Design review of the part built by this model. Coordinates are the model's own, in mm. Face numbers are marked on the shaded views. A direction names the side the tool comes from. Coordinates: 2 decimals unless noted, no trailing zeros. Loops run counter-clockwise (first coordinate to the right, second up) from the corner with the lowest first, then second, coordinate; pieces in that order, holes last. Notation, with made-up numbers: (27, 58) -> (48, 58) arc R12 ccw to (48, 81) -> close; hole circle Ø11 at (31, 33.25). An arc over 180 degrees is marked (long way). Answer in a Markdown table with one row per item.
```python
from build123d import *

# Parameters (mm, degrees)
BOSS_EXTRUDE1_DEPTH     = 3.25
SKETCH2_R               = 3.76
BOSS_EXTRUDE2_DEPTH     = 1.75
CUT_EXTRUDE1_DEPTH      = 8.895146188
CUT_EXTRUDE1_DEPTH_BACK = 8.895146188
SKETCH3_R               = 2.5


with BuildPart() as part:
    # Sketch1 → Boss-Extrude1 (new body)
    with BuildSketch(Plane(origin=(0, 0, 0), x_dir=(1, 0, 0), z_dir=(0, 1, 0))):
        Polygon((4, -2.309401077), (0, -4.618802154), (-4, -2.309401077), (-4, 2.309401077), (0, 4.618802154), (4, 2.309401077), align=None)
    extrude(amount=-BOSS_EXTRUDE1_DEPTH)

    # Sketch2 → Boss-Extrude2 (add)
    with BuildSketch(Plane(origin=(0, -3.25, 0), x_dir=(1, 0, 0), z_dir=(0, 1, 0))):
        with Locations(Location((0, 0, 0), (0, 0, 270))):
            Circle(SKETCH2_R)
    extrude(amount=-BOSS_EXTRUDE2_DEPTH)

    # Sketch3 → Cut-Extrude1 (cut, two sides: drawn at the far end of the back side and taken through both)
    with BuildSketch(Plane(origin=(0, 0, 0), x_dir=(1, 0, 0), z_dir=(0, 1, 0)).offset(-CUT_EXTRUDE1_DEPTH_BACK)):
        with Locations(Location((0, 0, 0), (0, 0, 270))):
            Circle(SKETCH3_R)
    extrude(amount=CUT_EXTRUDE1_DEPTH + CUT_EXTRUDE1_DEPTH_BACK, mode=Mode.SUBTRACT)


solid = part.part
```
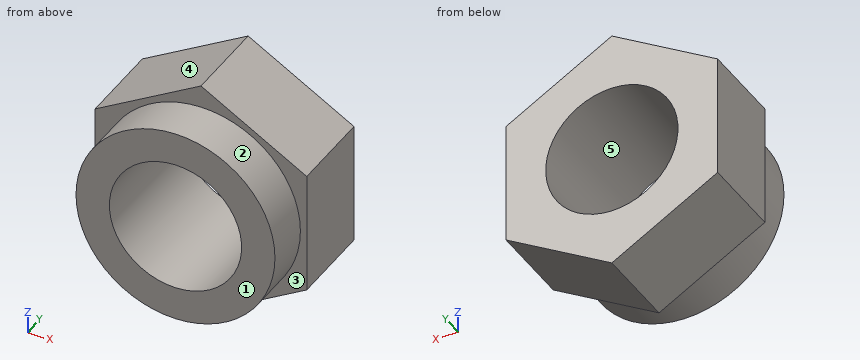
(1) To check wall thickness, follow probe 1 along X at (y, z) = (-3.85, 0); probe 2 along X at (y, z) = (-1.8, 0); probe 3 along Z at (x, y) = (-2, -1.95). State the ranges of each line that lie inside material, in increasing order.
Evaluation:
| item | result |
|---|---|
| probe 1 | x = -3.76 to -2.5, 2.5 to 3.76 |
| probe 2 | x = -4 to -2.5, 2.5 to 4 |
| probe 3 | z = -3.46 to -1.5, 1.5 to 3.46 |
(2) Draft analysis for pull direction X (two halves, no side actions). For the marked faces 3, 4 and 5, state which applies: pulls with the +X half, pulls with the -X half, needs draft (parallel to the pull), parting line crosses it, or undercut.
Evaluation:
| item | result |
|---|---|
| face 3 | needs draft |
| face 4 | pulls with the -X half |
| face 5 | undercut |
(3) Take a section at D-D on y = -4.65. Give the boundary of the cut face in (x, z).
Evaluation:
| item | result |
|---|---|
| outline | circle Ø7.52 at (0, 0); hole circle Ø5 at (0, 0) |
(4) For pin 1 (1 mm diameter, centred on y = -1, z = -3, fed in from +X), flat-tipped, find the tip position at first contact; note if it passes through.
Evaluation:
| item | result |
|---|---|
| pin 1 | stops at x = 3.67 |
(5) Take a section at A-A on z = 0. Give the boundary of the cut face in (x, y).
Evaluation:
| item | result |
|---|---|
| outline | (-4, -3.25) -> (-3.76, -3.25) -> (-3.76, -5) -> (-2.5, -5) -> (-2.5, 0) -> (-4, 0) -> close; (2.5, -5) -> (3.76, -5) -> (3.76, -3.25) -> (4, -3.25) -> (4, 0) -> (2.5, 0) -> close |
(6) Tool access review of the marked faces 1 and 2: name each direction out of +Z, -Z, +X, -X, +Y, -Y from which nothing blocks a thin tool from reaching the whole face with its end or side.
Evaluation:
| item | result |
|---|---|
| face 1 | +Z, -Z, +X, -X, -Y |
| face 2 | -Y |
(7) Take a section at C-C on y = -2.15. Give the boundary of the cut face in (x, z).
Evaluation:
| item | result |
|---|---|
| outline | (-4, -2.31) -> (0, -4.62) -> (4, -2.31) -> (4, 2.31) -> (0, 4.62) -> (-4, 2.31) -> close; hole circle Ø5 at (0, 0) |
(8) Take a section at B-B on x = -2.25. Give the boundary of the cut face in (y, z), and give its area (3 significant figures).
Evaluation:
| item | result |
|---|---|
| outline | (-5, -3.01) -> (-3.25, -3.01) -> (-3.25, -3.32) -> (0, -3.32) -> (0, -1.09) -> (-5, -1.09) -> close; (-5, 1.09) -> (0, 1.09) -> (0, 3.32) -> (-3.25, 3.32) -> (-3.25, 3.01) -> (-5, 3.01) -> close |
| area | 21.2 mm² |
